Can you work these out from the model? Positions are in its coordinate system, mm. Coordinates: 2 decimals unless noted, no trailing zeros. Order: outer loops, then holes, each group sorted by start corner. A loop starts at its lowest first (then second) coordinate and runs counter-clockwise, first axis right, second up. Notation, with made-up numbers: (-8.5, -30.75) -> (29.5, -30.75) arc R17 cw to (29.5, -24.75) -> close; hole circle Ø10 at (35, 33.25). An arc over 180 degrees is marked (long way). Write item = value, one per line.
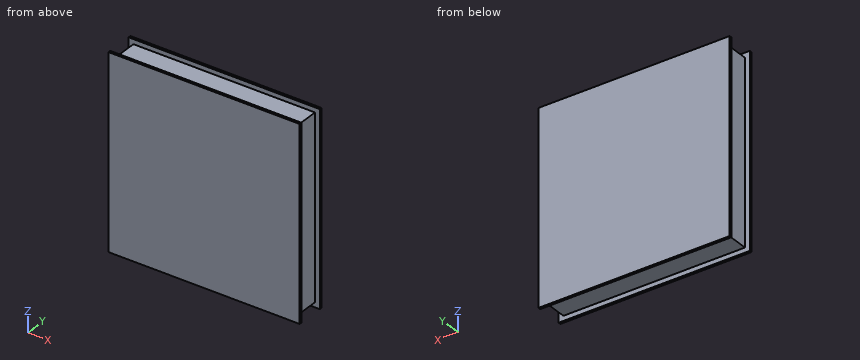
```python
from build123d import *

# Parameters (mm, degrees)
SKETCH1_W           = 10.0076
SKETCH1_H           = 10.0076
SKETCH1_W_2         = 9.4996
SKETCH1_H_2         = 9.4996
BOSS_EXTRUDE1_DEPTH = 0.127
SKETCH2_W           = 9.4996
SKETCH2_H           = 9.4996
BOSS_EXTRUDE2_DEPTH = 1.6002
SKETCH3_W           = 10.0076
SKETCH3_H           = 10.0076
SKETCH3_W_2         = 9.4996
SKETCH3_H_2         = 9.4996
BOSS_EXTRUDE3_DEPTH = 0.127


with BuildPart() as part:
    # Sketch1 → Boss-Extrude1 (new body)
    with BuildSketch(Plane(origin=(0, 0, 0), x_dir=(1, 0, 0), z_dir=(0, 1, 0))):
        with Locations((-0.7855503, 0.539979905)):
            Rectangle(SKETCH1_W, SKETCH1_H)
        with Locations((-0.7855503, 0.539979905)):
            Rectangle(SKETCH1_W_2, SKETCH1_H_2, mode=Mode.SUBTRACT)
    extrude(amount=BOSS_EXTRUDE1_DEPTH)

    # Sketch2 → Boss-Extrude2 (add)
    with BuildSketch(Plane(origin=(0, 0, 0), x_dir=(-1, 0, 0), z_dir=(0, -1, 0))):
        with Locations((0.7855503, 0.539979905)):
            Rectangle(SKETCH2_W, SKETCH2_H)
    extrude(amount=-BOSS_EXTRUDE2_DEPTH)

    # Sketch3 → Boss-Extrude3 (add)
    with BuildSketch(Plane(origin=(0, 1.6002, 0), x_dir=(1, 0, 0), z_dir=(0, 1, 0))):
        with Locations((-0.7855503, 0.539979905)):
            Rectangle(SKETCH3_W, SKETCH3_H)
        with Locations((-0.7855503, 0.539979905)):
            Rectangle(SKETCH3_W_2, SKETCH3_H_2, mode=Mode.SUBTRACT)
    extrude(amount=-BOSS_EXTRUDE3_DEPTH)


solid = part.part
```
Item 1: I'm going to push flat-ended pins straight in: P1, Ø0.7, axis at y = 1, z = 0, coming from the -X side; P2, Ø0.7, axis at y = 1, z = -0.5, coming from the +X side. Where does each tip first touch, or does it pass through?
A:
P1 = -5.54
P2 = 3.96
Item 2: If I drill on probe 1 along X at (y, z) = (0.8, -0.5); probe 2 along Z at (x, y) = (0, 1.3), over which ranges is the centre line in solid material (lowest first)?
A:
probe_1 = -5.54 to 3.96
probe_2 = -5.29 to 4.21
Item 3: I want a section at A-A, the plane z = 3. Please give me the cut outline in (x, y), plus the area to 3 significant figures.
A:
outline = (-5.79, 0) -> (4.22, 0) -> (4.22, 0.13) -> (3.96, 0.13) -> (3.96, 1.47) -> (4.22, 1.47) -> (4.22, 1.6) -> (-5.79, 1.6) -> (-5.79, 1.47) -> (-5.54, 1.47) -> (-5.54, 0.13) -> (-5.79, 0.13) -> close
area = 15.3 mm2
Item 4: I want a section at C-C, the plane y = 0.6. Please give me the cut outline in (x, z), plus the area to 3 significant figures.
A:
outline = (-5.54, -5.29) -> (3.96, -5.29) -> (3.96, 4.21) -> (-5.54, 4.21) -> close
area = 90.2 mm2
Item 5: I want a section at B-B, the plane x = 2.5. Please give me the cut outline in (y, z), plus the area to 3 significant figures.
A:
outline = (0, -5.54) -> (0.13, -5.54) -> (0.13, -5.29) -> (1.47, -5.29) -> (1.47, -5.54) -> (1.6, -5.54) -> (1.6, 4.46) -> (1.47, 4.46) -> (1.47, 4.21) -> (0.13, 4.21) -> (0.13, 4.46) -> (0, 4.46) -> close
area = 15.3 mm2
